Source: CAD feature listing. Evaluate the final solid. Frame: model axes, mm. A direction names the side the tool comes from. Round coordinates to 2 decimals unless told otherwise and drop trailing zeros. Order: outer loops, then holes, each group sorted by start corner. A loop starts at its lowest first (then second) coordinate and runs counter-clockwise, first axis right, second up. Notation, with made-up numbers: (79, 81) -> (115, 81) arc R31 cw to (115, 106) -> close; hole circle Ø6 at (45.25, 82). An arc over 180 degrees is marked (long way). Write item = value, one per line. Start each with the question number.
(1) Reachability of faces 4 (the face through (0, 20, 5)), 5 (the face through (0, -15, 33)) from +Z, -Z, +X, -X, +Y, -Y: full face, straight path, thin tool, end or side. Return the list, or none.
(2) Draft query along Y for faces 1 (the face through (18.03, 2.15, 32.95)), 2 (the face through (-0.59, 4.46, 4.93)), 3 (the face through (-1.245, -17.535, 41.998)). Return one class per face: released by +Y, released by -Y, zero draft, split by the parting line, or undercut.
(3) Contact query for flat-ended pins moving along their axis: pin 1 Ø2 at (x, z) = (8.5, 46.5) entering from +Y; pin 2 Ø10 at (x, y) = (-3, 1.5) entering from -Z; pin 3 Ø1 at (x, y) = (-9, 0.5) entering from +Z. Output: stop coordinate, or through.
(4) Cut plane C-C on x = -15. Return the cut outline in (y, z), then the cut area to 3 significant figures.
(5) Ray query, line 1 (Y direction, x = 0, z = 7.5); line 2 (X direction, y = -1, z = 36); line 3 (X direction, y = -18.65, z = 45). Return the intervals inside material, ascending.
(6) Cut plane D-D on z = 45. Return the cut outline in (x, y), then the cut area to 3 significant figures.
(7) Cut plane B-B on y = 0. Return the cut outline in (x, z).
(8) Cut plane A-A on x = 0. Return the cut outline in (y, z), then the cut area to 3 significant figures.
from build123d import *

# Parameters (mm, degrees)
CROQUIS1_W              = 40
CROQUIS1_H              = 40
CROQUIS1_R              = 4.5
SALIENTE_EXTRUIR1_DEPTH = 10
CROQUIS2_W              = 40
CROQUIS2_H              = 55
CROQUIS2_R              = 3.25
SALIENTE_EXTRUIR2_DEPTH = 5
SALIENTE_EXTRUIR3_DEPTH = 4
REDONDEO1_START         = -21
REDONDEO1_DEPTH         = 42


with BuildPart() as part:
    # Croquis1 → Saliente-Extruir1 (new body)
    with BuildSketch(Plane.XY):
        Rectangle(CROQUIS1_W, CROQUIS1_H)
        Circle(CROQUIS1_R, mode=Mode.SUBTRACT)
    extrude(amount=SALIENTE_EXTRUIR1_DEPTH)

    # Croquis2 → Saliente-Extruir2 (add)
    with BuildSketch(Plane.XZ.offset(20)):
        with Locations((0, 27.5)):
            Rectangle(CROQUIS2_W, CROQUIS2_H)
        with Locations(Location((0, 45, 0), (0, 0, 270))):
            Circle(CROQUIS2_R, mode=Mode.SUBTRACT)
    extrude(amount=-SALIENTE_EXTRUIR2_DEPTH)

    # Croquis3 → Saliente-Extruir3 (add)
    with BuildSketch(Plane(origin=(20, 0, 0), x_dir=(0, 0, -1), z_dir=(1, 0, 0))):
        Polygon((-55, -15), (-10, 20), (-10, -15), align=None)
    saliente_extruir3 = extrude(amount=-SALIENTE_EXTRUIR3_DEPTH)

    # Simetría1: Saliente-Extruir3 across plane
    add(saliente_extruir3.mirror(Plane(origin=(0, 0, 0), x_dir=(0, 0, 1), z_dir=(1, 0, 0))))

    # Redondeo1: read off the stored shape, not the designer's step
    # Redondeo1 outline → Redondeo1 (cut)
    with BuildSketch(Plane.YZ.offset(REDONDEO1_START)):
        with BuildLine():
            Line((20, 9.65689225), (20, 10))
            Line((20, 10), (19.789352217, 10.270832863))
            ThreePointArc((19.789352217, 10.270832863), (19.945873199, 9.981428675), (20, 9.65689225))
        make_face()
    extrude(amount=REDONDEO1_DEPTH, mode=Mode.SUBTRACT)


solid = part.part
Evaluation:
q1.face_4 = +Z, -Z, +X, -X, +Y
q1.face_5 = +Z, +Y
q2.face_1 = released by +Y
q2.face_2 = undercut
q2.face_3 = zero draft
q3.pin_1 = -15
q3.pin_2 = 0
q3.pin_3 = 10
q4.outline = (-20, 0) -> (20, 0) -> (20, 9.66) arc R1 ccw to (19.94, 10) -> (-15, 10) -> (-15, 55) -> (-20, 55) -> close
q4.area = 625 mm^2
q5.line_1 = -20 to -4.5, 4.5 to 20
q5.line_2 = -20 to -16, 16 to 20
q5.line_3 = -20 to -3.25, 3.25 to 20
q6.outline = (-20, -20) -> (-3.25, -20) -> (-3.25, -15) -> (-16, -15) -> (-16, -7.22) -> (-20, -7.22) -> close; (3.25, -20) -> (20, -20) -> (20, -7.22) -> (16, -7.22) -> (16, -15) -> (3.25, -15) -> close
q6.area = 230 mm^2
q7.outline = (-20, 0) -> (-4.5, 0) -> (-4.5, 10) -> (-16, 10) -> (-16, 35.71) -> (-20, 35.71) -> close; (4.5, 0) -> (20, 0) -> (20, 35.71) -> (16, 35.71) -> (16, 10) -> (4.5, 10) -> close
q8.outline = (-20, 0) -> (-4.5, 0) -> (-4.5, 10) -> (-15, 10) -> (-15, 41.75) -> (-20, 41.75) -> close; (-20, 48.25) -> (-15, 48.25) -> (-15, 55) -> (-20, 55) -> close; (4.5, 0) -> (20, 0) -> (20, 9.66) arc R1 ccw to (19.94, 10) -> (4.5, 10) -> close
q8.area = 502 mm^2
